Build history of the part. All positions in model axes, mm. Round coordinates to 2 decimals unless told otherwise and drop trailing zeros. Loops run counter-clockwise (first coordinate to the right, second up) from the corner with the lowest first, then second, coordinate; pieces in that order, holes last. Notation, with made-up numbers: (63.5, 69) - (88.5, 69) arc R5 ccw to (88.5, 73) - close; hole circle Ø4 at (89.5, 34). An arc over 180 degrees is marked (long way). Put each result on its own line as item: value. Start each with the question number.
from build123d import *

# Parameters (mm, degrees)
BOSS_EXTRUDE4_DEPTH            = 5
M6_CLEARANCE_HOLE1_D           = 6.6
M6_CLEARANCE_HOLE1_CSINK_D     = 6.65
M6_CLEARANCE_HOLE1_CSINK_ANGLE = 90
SKETCH10_R                     = 2.5
CUT_EXTRUDE1_DEPTH             = 5


with BuildPart() as part:
    # Sketch6 → Boss-Extrude4 (new body)
    with BuildSketch(Plane.XY):
        with BuildLine():
            ThreePointArc((37.730032203, 0), (51.79672204, 71.134128832), (77.049643457, 139.106373223))
            ThreePointArc((77.049643457, 139.106373223), (0, 260), (-77.049643457, 139.106373223))
            ThreePointArc((-77.049643457, 139.106373223), (-51.79672204, 71.134128832), (-37.730032203, 0))
            ThreePointArc((-37.730032203, 0), (0, -37.730032203), (37.730032203, 0))
        make_face()
    extrude(amount=BOSS_EXTRUDE4_DEPTH)

    # M6 Clearance Hole1 (through all)
    with Locations(Plane.XY.offset(5)):
        with Locations((0, 25), (25, 0), (0, -25), (-25, 0)):
            CounterSinkHole(M6_CLEARANCE_HOLE1_D / 2, M6_CLEARANCE_HOLE1_CSINK_D / 2, counter_sink_angle=M6_CLEARANCE_HOLE1_CSINK_ANGLE)

    # Sketch10 → Cut-Extrude1 (cut)
    with BuildSketch(Plane.XY.offset(5)):
        with Locations((-25, 175)):
            Circle(SKETCH10_R)
        with Locations((25, 175)):
            Circle(SKETCH10_R)
    extrude(amount=-CUT_EXTRUDE1_DEPTH, mode=Mode.SUBTRACT)


solid = part.part
Item 1: Two-plate mould, pull along Y, no slides. Class faces 1 (the cylindrical face through (-52.074, 72.112, 2.465)), 2 (the cylindrical face through (21.95, -1.26, 2.45)), 3 (the flat face through (-1, 146, 5)), 4 (the cylindrical face through (0.72, -28.22, 2.45)): pulls with the +Y half, pulls with the -Y half, needs draft (parallel to the pull), parting line crosses it, or undercut.
Item 2: Drop a flat-ended pin along its axis: pin 1 Ø2 at (y, z) = (52.5, 0.5) entering from +X. Give the stop position or say it passes through.
Item 3: Slice it at B-B (y = 25). Give the cut face in (x, z) (3 decimals), plus the area to 3 significant figures.
Item 4: Slice it at C-C (x = 68). Give the cut face in (y, z).
Item 5: Slice it at A-A (x = 0). Give the cut face in (y, z) (3 decimals), plus the area to 3 significant figures.
Item 6: Drill centre lines: probe 1 along Y at (x, z) = (25, 3.45); probe 2 along X at (y, z) = (0, 3.5); probe 3 along X at (y, z) = (-25, 1.7). Where is each one in solid material? Low to high. Write a range as [from, to].
Item 7: Slice it at D-D (y = 69.5). Give the cut face in (x, z), plus the area to 3 significant figures.
Computed values:
1. face 1: pulls with the -Y half
1. face 2: undercut
1. face 3: needs draft
1. face 4: undercut
2. pin 1: stops at x = 47.19
3. outline: (-41.327, 0) - (-3.3, 0) - (-3.3, 4.975) - (-3.325, 5) - (-41.327, 5) - close; (3.3, 0) - (41.327, 0) - (41.327, 5) - (3.325, 5) - (3.3, 4.975) - close
3. area: 380 mm^2
4. outline: (118.34, 0) - (226, 0) - (226, 5) - (118.34, 5) - close
5. outline: (-37.73, 0) - (-28.3, 0) - (-28.3, 4.975) - (-28.325, 5) - (-37.73, 5) - close; (-21.7, 0) - (21.7, 0) - (21.7, 4.975) - (21.675, 5) - (-21.675, 5) - (-21.7, 4.975) - close; (28.3, 0) - (260, 0) - (260, 5) - (28.325, 5) - (28.3, 4.975) - close
5. area: 1,420 mm^2
6. probe 1: y = [-28.26, -3.3], [3.3, 172.5], [177.5, 256.24]
6. probe 2: x = [-37.73, -28.3], [-21.7, 21.7], [28.3, 37.73]
6. probe 3: x = [-28.26, -3.3], [3.3, 28.26]
7. outline: (-51.34, 0) - (51.34, 0) - (51.34, 5) - (-51.34, 5) - close
7. area: 513 mm^2
